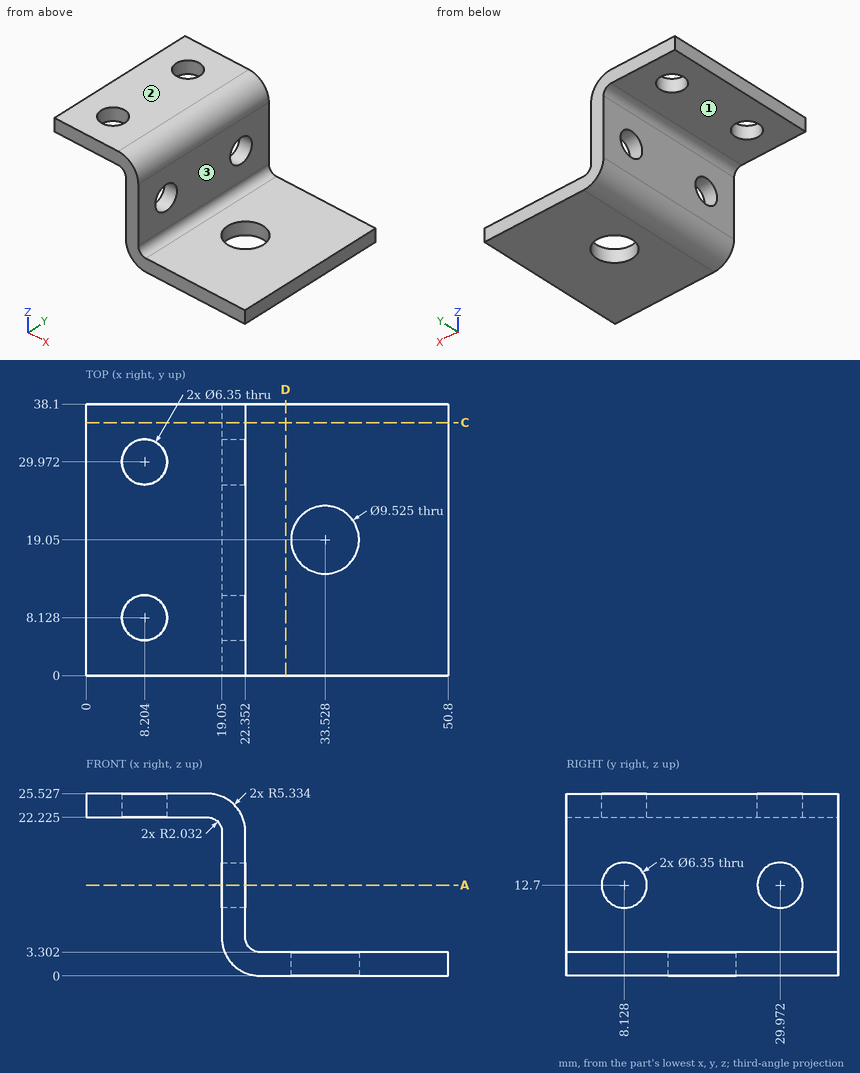
Answer from the drawing. Dimensions are ordinates in mm from the lowest x, y and z of the part. A direction names the side the tool comes from. Coordinates: 2 decimals unless noted, no trailing zeros. Order: outer loops, then holes, each group sorted by start corner. A loop starts at its lowest first (then second) coordinate and runs counter-clockwise, first axis right, second up. Notation, with made-up numbers: (74, 53) - (130, 53) arc R24 cw to (130, 89) - close; hole circle Ø5 at (48.25, 75.25). An arc over 180 degrees is marked (long way). Answer as a JSON object with one key per item and string values. Group by question number.
Item 1: Section A-A (z = 12.7) is taken. Give the vertices of the cut face in (x, y).
Item 2: Section C-C (y = 35.5) is taken. Give the vertices of the cut face in (x, z) (3 decimals).
Item 3: Flat-ended cylindrical pins translate along their axes: P1, Ø8.5, axis at y = 29.972, z = 12.7, coming from the -X side; P2, Ø10, axis at x = 27.5, z = 10, coming from the +Y side; P3, Ø12.5, axis at x = 33.528, y = 19.05, coming from the +Z side; P4, Ø13.5, axis at x = 7.5, y = 20, coming from the -Z side (3 decimals). Find the tip coordinate at first contact, or state that the pin passes through.
Item 4: Consider probe 1 along X at (y, z) = (6, 6); probe 2 along Y at (x, z) = (36, 2.25); probe 3 along Z at (x, y) = (8, 35) (3 decimals). Determine where each line is inside the solid, lowest interval first. Write a range as from..to.
Item 5: A tool of negligible diameter and unlimited length cuts with its end or side. For the marked faces 1, 2 and 3, from which of +Z, -Z, +X, -X, +Y, -Y can it reach the whole face along a straight path? Write none if from no direction.
Item 6: Section D-D (x = 28) is taken. Give the vertices of the cut face in (y, z).
Results are:
{
 "1": {"outline": "(19.05, 0) - (22.35, 0) - (22.35, 4.95) - (19.05, 4.95) - close; (19.05, 11.3) - (22.35, 11.3) - (22.35, 26.8) - (19.05, 26.8) - close; (19.05, 33.15) - (22.35, 33.15) - (22.35, 38.1) - (19.05, 38.1) - close"},
 "2": {"outline": "(0, 22.225) - (17.018, 22.225) arc R2.032 cw to (19.05, 20.193) - (19.05, 5.334) arc R5.334 ccw to (24.384, 0) - (50.8, 0) - (50.8, 3.302) - (24.384, 3.302) arc R2.032 cw to (22.352, 5.334) - (22.352, 20.193) arc R5.334 ccw to (17.018, 25.527) - (0, 25.527) - close"},
 "3": {"P1": "stops at x = 19.05", "P2": "passes through", "P3": "stops at z = 3.3", "P4": "stops at z = 22.225"},
 "4": {"probe 1": "x = 19.05..22.35", "probe 2": "y = 0..14.98, 23.12..38.1", "probe 3": "z = 22.225..25.527"},
 "5": {"face 1": "-Z, -X, +Y, -Y", "face 2": "+Z, +X, -X, +Y, -Y", "face 3": "+Z, +X, +Y, -Y"},
 "6": {"outline": "(0, 0) - (38.1, 0) - (38.1, 3.3) - (0, 3.3) - close"}
}
